The listing builds one solid part. Answer for the finished solid, in the listing's coordinates (mm). A direction names the side the tool comes from. Coordinates: 2 decimals unless noted, no trailing zeros. Order: outer loops, then holes, each group sorted by start corner. A loop starts at its lowest first (then second) coordinate and runs counter-clockwise, first axis right, second up. Notation, with made-up numbers: (25, -17) -> (56, -17) arc R27 ccw to (56, 12) -> close; hole circle Ø3 at (-1.5, 74.25). An arc over 180 degrees is marked (long way). Write item = value, one per line.
from build123d import *

# Parameters (mm, degrees)
F1_DEPTH  = 12.7
F5_R      = 3.302
F4_FACE_R = 5.2264022723
F6_DEPTH  = 6.35
F7_DEPTH  = 6.35
F8_DEPTH  = 6.35
F9_R      = 2.8667617308
F10_DEPTH = 6.35
F11_R     = 3.175


with BuildPart() as f1:
    # F0 (on Front) → F1 (new body, symmetric)
    with BuildSketch(Plane.XZ):
        with BuildLine():
            Line((27.0537398756, 6.9073382765), (-39.1415841877, 6.9073382765))
            ThreePointArc((-39.1415841877, 6.9073382765), (-49.8380616626, -0.7794862001), (-39.7171936929, -9.2097846791))
            Line((-39.7171936929, -9.2097846791), (27.0537398756, -9.2097846791))
            ThreePointArc((27.0537398756, -9.2097846791), (35.1123013534, -1.1512232013), (27.0537398756, 6.9073382765))
        make_face()
    extrude(amount=F1_DEPTH, both=True)

    # F3 (on Front) → F4 (revolve)
    with BuildSketch(Plane.XZ):
        with BuildLine():
            ThreePointArc((-19.0515599295, 6.0564640567), (-21.5885566512, 7.6841524566), (-23.0529304126, 10.3187931113))
            Line((-23.0529304126, 10.3187931113), (-25.4015599295, 10.3187931113))
            Line((-25.4015599295, 10.3187931113), (-25.4015599295, 6.0564640567))
            Line((-25.4015599295, 6.0564640567), (-19.0515599295, 6.0564640567))
        make_face()
    revolve(axis=Axis((-30.6279622018, 0, 0.5539879203), (0, 0, -1)))

    # F5 (on Top) + F4_face (on face) → F6 (cut)
    with BuildSketch(Plane.XY):
        with Locations((-31.2027800828, 0)):
            Circle(F5_R)
    with BuildSketch(Plane(origin=(-30.6279622018, 0, 6.9073382765), x_dir=(1, 0, 0), z_dir=(0, 0, 1))):
        Circle(F4_FACE_R)
    extrude(amount=-F6_DEPTH, mode=Mode.SUBTRACT)

    # F5 (on Top) → F7 (cut)
    with BuildSketch(Plane.XY):
        with Locations((-31.2027800828, 0)):
            Circle(F5_R)
    extrude(amount=-F7_DEPTH, mode=Mode.SUBTRACT)

    # F5 (on Top) → F8 (cut)
    with BuildSketch(Plane.XY):
        with Locations((-31.2027800828, 0)):
            Circle(F5_R)
    extrude(amount=-F8_DEPTH, mode=Mode.SUBTRACT)

    # F9 (on face) → F10 (cut)
    with BuildSketch(Plane.XY.offset(0.5573382765)):
        with Locations((-30.1966872066, 0)):
            Circle(F9_R)
    extrude(amount=-F10_DEPTH, mode=Mode.SUBTRACT)

    # F11
    f11_edges = [f1.edges().sort_by_distance(p)[0] for p in [
        (-6.043922, -12.7, 6.907338),
        (-6.043922, 12.7, 6.907338),
        (-49.838062, -12.7, -0.779486),
    ]]
    fillet(f11_edges, radius=F11_R)


solid = f1.part
Q1. A tool of negligible diameter and unlimited length cuts with its end or side. For faces 4 (the face through (-7, 0, -9.21)), 5 (the face through (-0.78, 11.75, 6)), 6 (the face through (-33.02, -1.09, 0.557)), 7 (the face through (-33.3, -0.5, 0)), 8 (the face through (-38, 8, 6.907)), from which of +Z, -Z, +X, -X, +Y, -Y can it reach the whole face along a straight path? Write none if from no direction.
The answers:
face_4 = -Z, +X, +Y, -Y
face_5 = +Z, +X, +Y
face_6 = +Z
face_7 = none
face_8 = +Z, +Y
Q2. Section B-B, the plane y = 0 is taken. Give the vertices of the cut face in (x, z), plus the area to 3 significant figures.
The answers:
outline = (-40.23, 7.15) arc R8.33 ccw (long way) to (-39.72, -9.21) -> (27.05, -9.21) arc R8.06 ccw to (27.05, 6.91) -> (-20.71, 6.91) arc R6.18 cw to (-23.05, 10.32) -> (-25.4, 10.32) -> (-25.4, 0.56) -> (-27.33, 0.56) -> (-27.33, -5.79) -> (-27.9, -5.79) -> (-27.9, -6.35) -> (-34.5, -6.35) -> (-34.5, 0) -> (-33.06, 0) -> (-33.06, 0.56) -> (-35.85, 0.56) -> (-35.85, 10.32) -> (-38.2, 10.32) arc R6.18 cw to start
area = 1,220 mm2
Q3. Section A-A, the plane x = 5 is taken. Give the vertices of the cut face in (y, z) (3 decimals), plus the area to 3 significant figures.
The answers:
outline = (-12.7, -6.035) arc R3.175 ccw to (-9.525, -9.21) -> (9.525, -9.21) arc R3.175 ccw to (12.7, -6.035) -> (12.7, 3.732) arc R3.175 ccw to (9.525, 6.907) -> (-9.525, 6.907) arc R3.175 ccw to (-12.7, 3.732) -> close
area = 401 mm2
Q4. Each of these flat-tipped pins is pushed along its axis until it touches: pin 1 Ø8.5 at (x, y) = (-31.2, 0) entering from +Z; pin 2 Ø1.5 at (y, z) = (2.5, 6.5) entering from -X; pin 3 Ø8 at (y, z) = (-10, 6) entering from +X. Where does it stop, or does it pass through?
The answers:
pin_1 = 0.56
pin_2 = -46.29
pin_3 = 34.46
Q5. The mould has two halves that part along Z. Classify faces 1 (the face through (-49.834, 1.432, -0.692)), 2 (the face through (-36.58, -11.75, 6)), 3 (the face through (-31, 0, -6.35)): released by +Z, released by -Z, zero draft, split by the parting line, or undercut.
The answers:
face_1 = split by the parting line
face_2 = released by +Z
face_3 = undercut
Q6. Find the intervals of material crossed by line 1 along X through (y, z) = (0, -0.75); line 2 along Z through (x, y) = (-11.5, -0.25); line 3 along Z through (x, y) = (-42, 10.5), in increasing order.
The answers:
line_1 = -49.84 to -34.5, -27.33 to 35.1
line_2 = -9.21 to 6.91
line_3 = -9.39 to 7.24
